The model under review builds one solid part; all positions refer to its coordinate system, in mm. A direction names the side the tool comes from. Round coordinates to 2 decimals unless told otherwise and drop trailing zeros.
```python
from build123d import *

# Parameters (mm, degrees)
SKETCH2_W                                  = 320
SKETCH2_H                                  = 160
BOSS_EXTRUDE1_DEPTH                        = 2
SKETCH3_R                                  = 1.6
CUT_EXTRUDE1_DEPTH                         = 7
CUT_EXTRUDE2_DEPTH                         = 12.5
MIRROR1_AT_THE_SECOND_PLANE_COPY_1_SKETC_R = 1.6
MIRROR1_AT_THE_SECOND_PLANE_COPY_1_DEPTH   = 7
MIRROR1_AT_THE_SECOND_PLANE_COPY_2_DEPTH   = 12.5
SKETCH4_W                                  = 8.5
SKETCH4_H                                  = 28
SKETCH4_W_2                                = 16
SKETCH4_H_2                                = 8
BOSS_EXTRUDE3_DEPTH                        = 10
SKETCH5_R                                  = 1.5
BOSS_EXTRUDE4_DEPTH                        = 2


with BuildPart() as part:
    # Sketch2 → Boss-Extrude1 (new body)
    with BuildSketch(Plane(origin=(0, 13, 0), x_dir=(1, 0, 0), z_dir=(0, 1, 0))):
        Rectangle(SKETCH2_W, SKETCH2_H)
    extrude(amount=BOSS_EXTRUDE1_DEPTH)

    # Sketch1 → Loft1 section 0
    with BuildSketch(Plane(origin=(0, 0, 0), x_dir=(1, 0, 0), z_dir=(0, 1, 0))):
        with BuildLine():
            Line((-158.5, -78.5), (158.5, -78.5))
            Line((158.5, -78.5), (158.5, 78.5))
            Line((158.5, 78.5), (-158.5, 78.5))
            Line((-158.5, 78.5), (-158.5, -78.5))
        make_face()
    # Sketch2_2 → Loft1 section 1
    with BuildSketch(Plane(origin=(0, 13, 0), x_dir=(1, 0, 0), z_dir=(0, 1, 0))):
        with BuildLine():
            Line((160, -80), (-160, -80))
            Line((-160, -80), (-160, 80))
            Line((-160, 80), (160, 80))
            Line((160, 80), (160, -80))
        make_face()
    loft()

    # Sketch3 → Cut-Extrude1 (cut)
    with BuildSketch(Plane.XZ):
        with Locations(Location((0, 70, 0), (0, 0, 270))):
            Circle(SKETCH3_R)
        with Locations(Location((-152, 70, 0), (0, 0, 270))):
            Circle(SKETCH3_R)
    cut_extrude1 = extrude(amount=-CUT_EXTRUDE1_DEPTH, mode=Mode.SUBTRACT)

    # Sketch3_4 → Cut-Extrude2 (cut)
    with BuildSketch(Plane.XZ):
        with BuildLine():
            Line((-150.2, 19.75), (-150.2, 0))
            Line((-150.2, 0), (-9, 0))
            Line((-9, 0), (-9, 67.9))
            Line((-9, 67.9), (-142.1, 67.9))
            ThreePointArc((-142.1, 67.9), (-145.281980515, 66.581980515), (-146.6, 63.4))
            Line((-146.6, 63.4), (-146.6, 22.75))
            Line((-146.6, 22.75), (-150.2, 19.75))
        make_face()
    cut_extrude2 = extrude(amount=-CUT_EXTRUDE2_DEPTH, mode=Mode.SUBTRACT)

    # Mirror1: Cut-Extrude1, Cut-Extrude2 across plane
    add(cut_extrude1.mirror(Plane.XY), mode=Mode.SUBTRACT)
    add(cut_extrude2.mirror(Plane.XY), mode=Mode.SUBTRACT)

    # Mirror1 at the second plane: Cut-Extrude1, Cut-Extrude2 across plane
    add(cut_extrude1.mirror(Plane(origin=(0, 0, 0), x_dir=(0, 0, 1), z_dir=(1, 0, 0))), mode=Mode.SUBTRACT)
    add(cut_extrude2.mirror(Plane(origin=(0, 0, 0), x_dir=(0, 0, 1), z_dir=(1, 0, 0))), mode=Mode.SUBTRACT)

    # Mirror1 at the second plane copy 1 sketc → Mirror1 at the second plane copy 1 (cut)
    with BuildSketch(Plane(origin=(0, 0, 0), x_dir=(-1, 0, 0), z_dir=(0, -1, 0))):
        with Locations(Location((0, 70, 0), (0, 0, 270))):
            Circle(MIRROR1_AT_THE_SECOND_PLANE_COPY_1_SKETC_R)
        with Locations(Location((-152, 70, 0), (0, 0, 270))):
            Circle(MIRROR1_AT_THE_SECOND_PLANE_COPY_1_SKETC_R)
    extrude(amount=-MIRROR1_AT_THE_SECOND_PLANE_COPY_1_DEPTH, mode=Mode.SUBTRACT)

    # Mirror1 at the second plane copy 2 sketc → Mirror1 at the second plane copy 2 (cut)
    with BuildSketch(Plane(origin=(0, 0, 0), x_dir=(-1, 0, 0), z_dir=(0, -1, 0))):
        with BuildLine():
            Line((-150.2, 19.75), (-150.2, 0))
            Line((-150.2, 0), (-9, 0))
            Line((-9, 0), (-9, 67.9))
            Line((-9, 67.9), (-142.1, 67.9))
            ThreePointArc((-142.1, 67.9), (-145.281980515, 66.581980515), (-146.6, 63.4))
            Line((-146.6, 63.4), (-146.6, 22.75))
            Line((-146.6, 22.75), (-150.2, 19.75))
        make_face()
    extrude(amount=-MIRROR1_AT_THE_SECOND_PLANE_COPY_2_DEPTH, mode=Mode.SUBTRACT)

    # Sketch4 → Boss-Extrude3 (add)
    with BuildSketch(Plane.XZ.offset(-12.5)):
        with Locations((-112.45, 0)):
            Rectangle(SKETCH4_W, SKETCH4_H)
        with Locations((31, 13)):
            Rectangle(SKETCH4_W_2, SKETCH4_H_2)
        with Locations((112.45, 0)):
            Rectangle(SKETCH4_W, SKETCH4_H)
    extrude(amount=BOSS_EXTRUDE3_DEPTH)

    # Sketch5 → Boss-Extrude4 (add)
    with BuildSketch(Plane.XZ):
        with Locations(Location((-110, 71.5, 0), (0, 0, 270))):
            Circle(SKETCH5_R)
        with Locations(Location((110, -71.5, 0), (0, 0, 270))):
            Circle(SKETCH5_R)
    extrude(amount=BOSS_EXTRUDE4_DEPTH)


solid = part.part
```
(1) For faces 1 (the flat face through (112, 8, -14)), 2 (the flat face through (-2, 15, -1)), list the 3-axis set-ups (+Z, -Z, +X, -X, +Y, -Y) from which the entire face can be reached by the end or side of a thin tool; tool diameter is ignored.
Data:
face 1: -Y
face 2: +Z, -Z, +X, -X, +Y
(2) To check wall thickness, follow probe 1 along X at (y, z) = (0.25, -14.5); probe 2 along X at (y, z) = (3.5, -70); probe 3 along X at (y, z) = (3.5, 22.5). State the ranges of each line that lie inside material, in increasing order.
Data:
probe 1: x = -158.53 to -150.2, -9 to 9, 150.2 to 158.53
probe 2: x = -158.9 to -153.6, -150.4 to -1.6, 1.6 to 150.4, 153.6 to 158.9
probe 3: x = -158.9 to -146.9, -9 to 9, 146.9 to 158.9
(3) Insertion check: pin 1 (4 mm diameter, centred on x = -43.5, y = 4.5, fed in from +Z); pin 2 (2.5 mm diameter, centred on x = -0.5, z = 69.5, fed in from -Y); pin 3 (8 mm diameter, centred on x = -33.5, y = 1, fed in from +Z). Each pin has a flat end and moves straight along its axis. Give the tip position at first contact, or say it passes through.
Data:
pin 1: stops at z = 79.25
pin 2: stops at y = 0
pin 3: stops at z = 79.08
(4) Draft analysis for pull direction Z (two halves, no side actions). For faces 3 (the flat face through (-150.2, 6, 0)), 4 (the flat face through (0, 0, 1)), state which applies: pulls with the +Z half, pulls with the -Z half, needs draft (parallel to the pull), parting line crosses it, or undercut.
Data:
face 3: undercut
face 4: needs draft
